Job drawing, mm, ordinate dimensions from the low corner. One solid piece. Give positions to 0.01 mm unless a question says otherwise; leave off trailing zeros. Order: outer loops, then holes, each group sorted by start corner. A loop starts at its lowest first (then second) coordinate and runs counter-clockwise, first axis right, second up.
1. Slice it at B-B on z = 5.5. List the corners of the cut face in (x, y).
2. Drop flat-ended pins along their axis: pin 1 Ø3.5 at (x, z) = (36.21, 5.5) entering from -Y; pin 2 Ø4 at (x, z) = (64, 7.5) entering from -Y. Give the stop position or say it passes through.
3. Probe line 1 (X direction, y = 3.45, z = 5.5); line 2 (Z direction, x = 51, y = 0.8); line 3 (X direction, y = 3.8, z = 7) (1 decimal). List the from-to ranges inside material, lowest first.
4. Slice it at D-D on x = 46. List the corners of the cut face in (y, z).
5. Slice it at A-A on x = 6. List the corners of the cut face in (y, z).
6. Slice it at C-C on y = 1.1. List the corners of the cut face in (x, z).
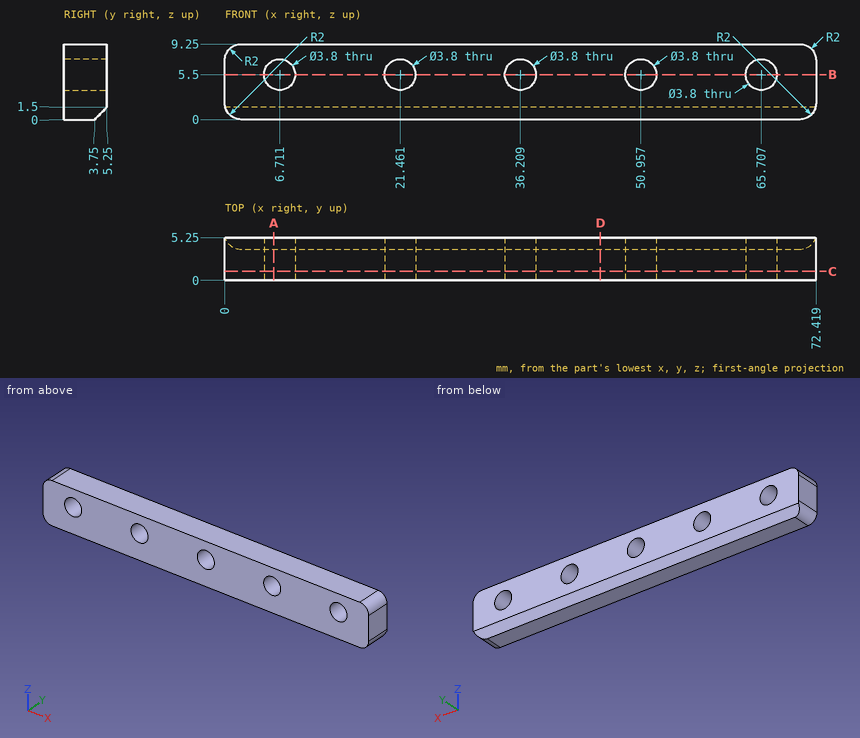
Data:
1. outline: (0, 0) - (4.81, 0) - (4.81, 5.25) - (0, 5.25) - close; (8.61, 0) - (19.56, 0) - (19.56, 5.25) - (8.61, 5.25) - close; (23.36, 0) - (34.31, 0) - (34.31, 5.25) - (23.36, 5.25) - close; (38.11, 0) - (49.06, 0) - (49.06, 5.25) - (38.11, 5.25) - close; (52.86, 0) - (63.81, 0) - (63.81, 5.25) - (52.86, 5.25) - close; (67.61, 0) - (72.42, 0) - (72.42, 5.25) - (67.61, 5.25) - close
2. pin 1: passes through
2. pin 2: stops at y = 0
3. line 1: x = 0 to 4.81, 8.61 to 19.56, 23.36 to 34.31, 38.11 to 49.06, 52.86 to 63.81, 67.61 to 72.42
3. line 2: z = 0 to 3.6, 7.4 to 9.25
3. line 3: x = 0 to 5.5, 7.9 to 20.3, 22.6 to 35, 37.4 to 49.8, 52.1 to 64.5, 66.9 to 72.4
4. outline: (0, 0) - (3.75, 0) - (5.25, 1.5) - (5.25, 9.25) - (0, 9.25) - close
5. outline: (0, 0) - (3.75, 0) - (5.25, 1.5) - (5.25, 3.74) - (0, 3.74) - close; (0, 7.26) - (5.25, 7.26) - (5.25, 9.25) - (0, 9.25) - close
6. outline: (0, 2) arc R2 ccw to (2, 0) - (70.42, 0) arc R2 ccw to (72.42, 2) - (72.42, 7.25) arc R2 ccw to (70.42, 9.25) - (2, 9.25) arc R2 ccw to (0, 7.25) - close; hole circle Ø3.8 at (6.71, 5.5); hole circle Ø3.8 at (21.46, 5.5); hole circle Ø3.8 at (36.21, 5.5); hole circle Ø3.8 at (50.96, 5.5); hole circle Ø3.8 at (65.71, 5.5)
